Source: CAD feature listing. Evaluate the final solid. Frame: model axes, mm. A direction names the side the tool comes from. Give positions to 0.01 mm unless a question says otherwise; leave off trailing zeros. Loops run counter-clockwise (first coordinate to the right, second up) from the corner with the lowest first, then second, coordinate; pieces in that order, holes last.
```python
from build123d import *

# Parameters (mm, degrees)
SKETCH1_W           = 66.04
SKETCH1_H           = 77.47
BOSS_EXTRUDE1_DEPTH = 30.1625
SKETCH2_W           = 64.21628
SKETCH2_H           = 77.47
CUT_EXTRUDE2_DEPTH  = 29.21
FILLET1_R           = 2.54
FILLET2_R           = 2.54
FILLET3_R           = 2.54
FILLET4_R           = 2.54
SKETCH5_R           = 2.54
CUT_EXTRUDE3_DEPTH  = 94.650885895


with BuildPart() as part:
    # Sketch1 → Boss-Extrude1 (new body)
    with BuildSketch(Plane.XY):
        with Locations((54.726493431, 20.420983827)):
            Rectangle(SKETCH1_W, SKETCH1_H)
    extrude(amount=BOSS_EXTRUDE1_DEPTH)

    # Sketch2 → Cut-Extrude2 (cut)
    with BuildSketch(Plane.XY.offset(30.1625)):
        with Locations((54.726493431, 20.420983827)):
            Rectangle(SKETCH2_W, SKETCH2_H)
    extrude(amount=-CUT_EXTRUDE2_DEPTH, mode=Mode.SUBTRACT)

    # Fillet1
    fillet1_edges = [part.edges().sort_by_distance(p)[0] for p in [
        (21.706493431, 20.420983827, 0),
    ]]
    fillet(fillet1_edges, radius=FILLET1_R)

    # Fillet2
    fillet2_edges = [part.edges().sort_by_distance(p)[0] for p in [
        (87.746493431, 20.420983827, 0),
    ]]
    fillet(fillet2_edges, radius=FILLET2_R)

    # Fillet3
    fillet3_edges = [part.edges().sort_by_distance(p)[0] for p in [
        (22.618353431, 20.420983827, 0.9525),
    ]]
    fillet(fillet3_edges, radius=FILLET3_R)

    # Fillet4
    fillet4_edges = [part.edges().sort_by_distance(p)[0] for p in [
        (86.834633431, 20.420983827, 0.9525),
    ]]
    fillet(fillet4_edges, radius=FILLET4_R)

    # Sketch5 → Cut-Extrude3 (cut, through all)
    with BuildSketch(Plane.ZY.offset(-21.706493431)):
        with Locations(Location((14.9225, 48.995983827, 0), (0, 0, 270))):
            Circle(SKETCH5_R)
    extrude(amount=-CUT_EXTRUDE3_DEPTH, mode=Mode.SUBTRACT)


solid = part.part
```
(1) Ray query, line 1 along X through (y, z) = (10, 27); line 2 along Z through (x, y) = (37.5, -2.5). Return the intervals inside material, ascending.
A:
line 1: x = 21.71 to 22.62, 86.83 to 87.75
line 2: z = 0 to 0.95
(2) Section C-C, the plane y = 20.5. Return the cut outline in (x, z).
A:
outline: (21.71, 2.54) arc R2.54 ccw to (24.25, 0) - (85.21, 0) arc R2.54 ccw to (87.75, 2.54) - (87.75, 30.16) - (86.83, 30.16) - (86.83, 3.49) arc R2.54 cw to (84.29, 0.95) - (25.16, 0.95) arc R2.54 cw to (22.62, 3.49) - (22.62, 30.16) - (21.71, 30.16) - close
(3) Section B-B, the plane z = 6.5. Return the cut outline in (x, y).
A:
outline: (21.71, -18.31) - (22.62, -18.31) - (22.62, 59.16) - (21.71, 59.16) - close; (86.83, -18.31) - (87.75, -18.31) - (87.75, 59.16) - (86.83, 59.16) - close
(4) Section A-A, the plane y = 49. Return the cut outline in (x, z), then the cut area to 3 significant figures.
A:
outline: (21.71, 2.54) arc R2.54 ccw to (24.25, 0) - (85.21, 0) arc R2.54 ccw to (87.75, 2.54) - (87.75, 12.38) - (86.83, 12.38) - (86.83, 3.49) arc R2.54 cw to (84.29, 0.95) - (25.16, 0.95) arc R2.54 cw to (22.62, 3.49) - (22.62, 12.38) - (21.71, 12.38) - close; (21.71, 17.46) - (22.62, 17.46) - (22.62, 30.16) - (21.71, 30.16) - close; (86.83, 17.46) - (87.75, 17.46) - (87.75, 30.16) - (86.83, 30.16) - close
area: 107 mm2
(5) First-contact query: pin 1 (4.5 mm diameter, centred on y = 49, z = 14.92, fed in from -X); pin 2 (5 mm diameter, centred on x = 56.5, y = -5.5, fed in from +Z). Flat tips, straight axial feed; report the tip coordinate or a pass-through.
A:
pin 1: passes through
pin 2: stops at z = 0.95
(6) Mould query, pull axis X, two halves, no side actions, for faces 1 (the flat face through (21.706, 20, 16)), 2 (the cylindrical face through (23.34, 20.96, 1.72)), 3 (the cylindrical face through (87.284, 46.573, 15.685)), 4 (the flat face through (87.746, 20, 16)). Classes: pulls with the +X half, pulls with the -X half, needs draft (parallel to the pull), parting line crosses it, or undercut.
A:
face 1: pulls with the -X half
face 2: undercut
face 3: needs draft
face 4: pulls with the +X half
(7) Section D-D, the plane x = 82. Return the cut outline in (y, z), then the cut area to 3 significant figures.
A:
outline: (-18.31, 0) - (59.16, 0) - (59.16, 0.95) - (-18.31, 0.95) - close
area: 73.8 mm2
(8) Reachability of faces 5 (the flat face through (54.6, 59.156, 0.5)), 6 (the flat face through (86.835, 20, 17)) from +Z, -Z, +X, -X, +Y, -Y: full face, straight path, thin tool, end or side. Return the list, or none.
A:
face 5: +Z, -Z, +X, -X, +Y
face 6: +Z, +Y, -Y
